Verification items for this drawing (mm, ordinates from the low corner). Round coordinates to 2 decimals unless told otherwise and drop trailing zeros. Loops run counter-clockwise (first coordinate to the right, second up) from the corner with the lowest first, then second, coordinate; pieces in that order, holes last. Notation, with made-up numbers: (88.25, 52.5) - (141.25, 52.5) arc R17 cw to (141.25, 59.5) - close; hole circle Ø7 at (-26.75, -7). An arc over 180 degrees is marked (long way). Answer in a Markdown table with one row per item. Add a question column.
(1) Cross-section at A-A on z = 127. Enter the section's corners in (x, y), then the cut area to 3 significant figures.
(2) Cross-section at B-B on x = 114.3. Enter the section's corners in (y, z).
(3) Gauge pin test, flat ends, axial feed: pin 1 (1.9 mm diameter, centred on y = 4, z = 43.5, fed in from +X); pin 2 (1 mm diameter, centred on x = 48, y = 1.5, fed in from +Z); pin 3 (2.5 mm diameter, centred on x = 38.76, z = 37.21, fed in from -Y); pin 4 (3 mm diameter, centred on x = 59.5, y = 2, fed in from +Z). Record the tip position at first contact, or that the pin passes through.
(4) Cross-section at C-C on y = 2.75. Enter the section's corners in (x, z).
(5) Cross-section at D-D on z = 112.5. Enter the section's corners in (x, y), then the cut area to 3 significant figures.
(6) Thickness scan on line 1 along X through (y, z) = (1.5, 37); line 2 along X through (y, z) = (4.5, 62.5) (1 decimal); line 3 along X through (y, z) = (5.75, 127.5) (1 decimal). Record the ranges inside material, lowest first.
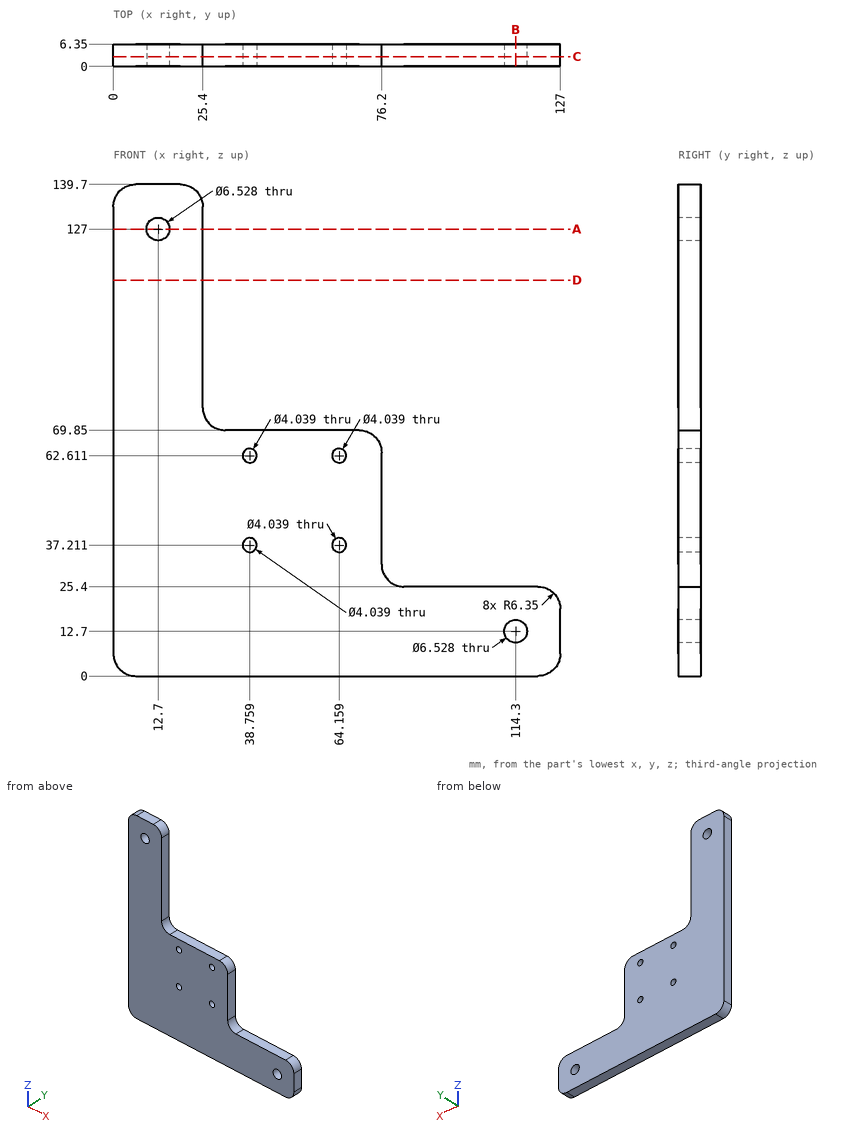
Answers:
| question | item | result |
|---|---|---|
| 1 | outline | (0, 0) - (9.44, 0) - (9.44, 6.35) - (0, 6.35) - close; (15.96, 0) - (25.4, 0) - (25.4, 6.35) - (15.96, 6.35) - close |
| 1 | area | 120 mm^2 |
| 2 | outline | (0, 0) - (6.35, 0) - (6.35, 9.44) - (0, 9.44) - close; (0, 15.96) - (6.35, 15.96) - (6.35, 25.4) - (0, 25.4) - close |
| 3 | pin 1 | stops at x = 76.2 |
| 3 | pin 2 | stops at z = 69.85 |
| 3 | pin 3 | passes through |
| 3 | pin 4 | stops at z = 69.85 |
| 4 | outline | (0, 6.35) arc R6.35 ccw to (6.35, 0) - (120.65, 0) arc R6.35 ccw to (127, 6.35) - (127, 19.05) arc R6.35 ccw to (120.65, 25.4) - (82.55, 25.4) arc R6.35 cw to (76.2, 31.75) - (76.2, 63.5) arc R6.35 ccw to (69.85, 69.85) - (31.75, 69.85) arc R6.35 cw to (25.4, 76.2) - (25.4, 133.35) arc R6.35 ccw to (19.05, 139.7) - (6.35, 139.7) arc R6.35 ccw to (0, 133.35) - close; hole circle Ø6.53 at (12.7, 127); hole circle Ø4.04 at (38.76, 37.21); hole circle Ø4.04 at (38.76, 62.61); hole circle Ø4.04 at (64.16, 37.21); hole circle Ø4.04 at (64.16, 62.61); hole circle Ø6.53 at (114.3, 12.7) |
| 5 | outline | (0, 0) - (25.4, 0) - (25.4, 6.35) - (0, 6.35) - close |
| 5 | area | 161 mm^2 |
| 6 | line 1 | x = 0 to 36.75, 40.77 to 62.15, 66.17 to 76.2 |
| 6 | line 2 | x = 0 to 36.7, 40.8 to 62.1, 66.2 to 76.2 |
| 6 | line 3 | x = 0 to 9.5, 15.9 to 25.4 |
